```python
from build123d import *

# Parameters (mm, degrees)
BOSS_EXTRUDE1_DEPTH = 3
BOSS_EXTRUDE2_DEPTH = 3
BOSS_EXTRUDE3_DEPTH = 10
FILLET1_R           = 10
FILLET2_R           = 1
CHAMFER1_SIZE       = 1
CHAMFER2_SIZE       = 0.5
FILLET4_R           = 0.5


with BuildPart() as part:
    # Sketch1 → Boss-Extrude1 (new body)
    with BuildSketch(Plane.XY):
        Polygon((55, 10), (55, -10), (24.791261432, -15), (-24.85397009, -15), (-55, -10), (-55, 10), (-24.85397009, 15), (24.791261432, 15), align=None)
        Polygon((-24.689236015, 13), (-53, 8.304395957), (-53, -8.304395957), (-24.689236015, -13), (24.626864724, -13), (53, -8.303819918), (53, 8.303819918), (24.626864724, 13), align=None, mode=Mode.SUBTRACT)
    extrude(amount=-BOSS_EXTRUDE1_DEPTH)

    # Sketch3 → Boss-Extrude2 (add)
    with BuildSketch(Plane.XY):
        Polygon((-53, 8.304395957), (-53, -8.304395957), (-24.689236015, -13), (24.626864724, -13), (53, -8.303819918), (53, 8.303819918), (24.626864724, 13), (-24.689236015, 13), align=None)
    extrude(amount=-BOSS_EXTRUDE2_DEPTH)

    # Sketch1_4 → Boss-Extrude3 (add)
    with BuildSketch(Plane.XY):
        Polygon((55, 10), (55, -10), (24.791261432, -15), (-24.85397009, -15), (-55, -10), (-55, 10), (-24.85397009, 15), (24.791261432, 15), align=None)
        Polygon((-24.689236015, 13), (-53, 8.304395957), (-53, -8.304395957), (-24.689236015, -13), (24.626864724, -13), (53, -8.303819918), (53, 8.303819918), (24.626864724, 13), align=None, mode=Mode.SUBTRACT)
    extrude(amount=BOSS_EXTRUDE3_DEPTH)

    # Fillet1
    fillet1_edges = [part.edges().sort_by_distance(p)[0] for p in [
        (24.791261432, -15, 3.5),
        (-24.85397009, -15, 3.5),
        (-24.85397009, 15, 3.5),
        (24.791261432, 15, 3.5),
        (-24.689236015, 13, 5),
        (24.626864724, 13, 5),
        (24.626864724, -13, 5),
        (-24.689236015, -13, 5),
    ]]
    fillet(fillet1_edges, radius=FILLET1_R)

    # Fillet2
    fillet2_edges = [part.edges().sort_by_distance(p)[0] for p in [
        (55, -10, 3.5),
        (-55, -10, 3.5),
        (-55, 10, 3.5),
        (55, 10, 3.5),
        (-53, 8.304395957, 5),
        (53, 8.303819918, 5),
        (53, -8.303819918, 5),
        (-53, -8.304395957, 5),
    ]]
    fillet(fillet2_edges, radius=FILLET2_R)

    # Chamfer1
    chamfer1_edges = [part.edges().sort_by_distance(p)[0] for p in [
        (-0.03051091, -15, -3),
        (-39.915081836, -12.501974258, -3),
        (-39.915081836, 12.501974258, -3),
        (-0.03051091, 15, -3),
        (-24.851190202, -14.966249987, -3),
        (-24.851190202, 14.966249987, -3),
        (24.78849853, 14.966387387, -3),
        (24.78849853, -14.966387387, -3),
        (55, 0, -3),
        (39.88275267, 12.50213151, -3),
        (39.88275267, -12.50213151, -3),
        (-55, 0, -3),
        (-54.762766018, -9.79887255, -3),
        (-54.762766018, 9.79887255, -3),
        (54.762657657, -9.798712323, -3),
        (54.762657657, 9.798712323, -3),
    ]]
    chamfer(chamfer1_edges, length=CHAMFER1_SIZE)

    # Chamfer2
    chamfer2_edges = [part.edges().sort_by_distance(p)[0] for p in [
        (-0.03051091, -15, 10),
        (-0.03051091, 15, 10),
        (-39.915081836, 12.501974258, 10),
        (-39.915081836, -12.501974258, 10),
        (-24.851190202, -14.966249987, 10),
        (-24.851190202, 14.966249987, 10),
        (24.78849853, 14.966387387, 10),
        (24.78849853, -14.966387387, 10),
        (55, 0, 10),
        (39.88275267, -12.50213151, 10),
        (39.88275267, 12.50213151, 10),
        (-55, 0, 10),
        (-54.762766018, -9.79887255, 10),
        (-54.762766018, 9.79887255, 10),
        (54.762657657, -9.798712323, 10),
        (54.762657657, 9.798712323, 10),
    ]]
    chamfer(chamfer2_edges, length=CHAMFER2_SIZE)

    # Fillet4
    fillet4_edges = [part.edges().sort_by_distance(p)[0] for p in [
        (-38.832714799, 10.654172237, 10),
        (-0.030342226, 13, 10),
        (-0.030342226, -13, 10),
        (-38.832714799, -10.654172237, 10),
        (24.624101823, -12.966387387, 10),
        (24.624101823, 12.966387387, 10),
        (-24.686456127, 12.966249987, 10),
        (-24.686456127, -12.966249987, 10),
        (38.800554316, 10.654041469, 10),
        (53, 0, 10),
        (38.800554316, -10.654041469, 10),
        (-53, 0, 10),
        (52.762657657, -8.10253224, 10),
        (52.762657657, 8.10253224, 10),
        (-52.762766018, 8.103268507, 10),
        (-52.762766018, -8.103268507, 10),
    ]]
    fillet(fillet4_edges, radius=FILLET4_R)


solid = part.part
```
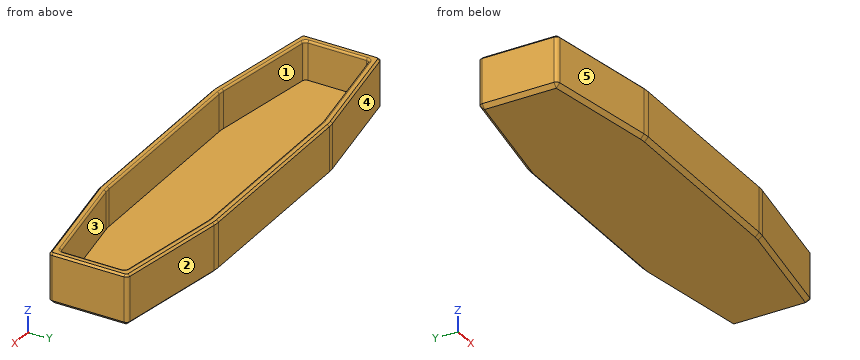
Build history of the part. All positions in model axes, mm. Face numbers are marked on the shaded views. A direction names the side the tool comes from. Round coordinates to 2 decimals unless told otherwise and drop trailing zeros. Order: outer loops, then holes, each group sorted by start corner. A loop starts at its lowest first (then second) coordinate and runs counter-clockwise, first axis right, second up. Notation, with made-up numbers: (3.5, 68) -> (59.5, 68) arc R22 ccw to (59.5, 83) -> close; hole circle Ø10 at (-21.5, 47.25). An arc over 180 degrees is marked (long way). Answer in a Markdown table with one row per item.
1) Which spindle directions (+Z, -Z, +X, -X, +Y, -Y) get a long thin tool onto all of the face, cutting with end or side? Do the marked faces 1 and 2. Say none if no direction does.
Values:
| item | result |
|---|---|
| face 1 | +Z |
| face 2 | +Z, -Z, +X, +Y |
2) Band-saw the part on C-C on y = 1.75. Give the cut face in (x, z).
Values:
| item | result |
|---|---|
| outline | (-55, -2) -> (-54, -3) -> (54, -3) -> (55, -2) -> (55, 9.5) -> (54.5, 10) -> (53.5, 10) arc R0.5 ccw to (53, 9.5) -> (53, 0) -> (-53, 0) -> (-53, 9.5) arc R0.5 ccw to (-53.5, 10) -> (-54.5, 10) -> (-55, 9.5) -> close |
3) Wall check: L1, parallel to Y at x = -4, z = 3.75; L2, parallel to X at y = -6.75, z = 0.75; L3, parallel to Z at x = 48, y = -5.5. Give the ranges that are in metal, low to high.
Values:
| item | result |
|---|---|
| L1 | -15 to -13, 13 to 15 |
| L2 | -55 to -53, 53 to 55 |
| L3 | -3 to 0 |
4) Mould opens along Y. For the marked faces 3, 4 and 5 say: released by +Y, released by -Y, zero draft, split by the parting line, or undercut.
Values:
| item | result |
|---|---|
| face 3 | undercut |
| face 4 | released by +Y |
| face 5 | released by -Y |
5) Band-saw the part on B-B on x = 1.5. Give the cut face in (y, z).
Values:
| item | result |
|---|---|
| outline | (-15, -2) -> (-14, -3) -> (14, -3) -> (15, -2) -> (15, 9.5) -> (14.5, 10) -> (13.5, 10) arc R0.5 ccw to (13, 9.5) -> (13, 0) -> (-13, 0) -> (-13, 9.5) arc R0.5 ccw to (-13.5, 10) -> (-14.5, 10) -> (-15, 9.5) -> close |
6) Pin check, flat tip, straight feed: P1, Ø2, axis at y = 10.5, z = 3, coming from the -X side. Stop position of the tip, or through.
Values:
| item | result |
|---|---|
| P1 | x = -54.94 |
